Autodesk Inventor part; units mm, degrees
ref_plane "YZ Plane" through (0, 0, 0) normal (1, 0, 0) x (0, 1, 0)
ref_plane "XZ Plane" through (0, 0, 0) normal (0, 1, 0) x (-1, 0, 0)
ref_plane "XY Plane" through (0, 0, 0) normal (0, 0, 1) x (1, 0, 0)
sketch "Sketch1" plane through (0, 0, 0) normal (0, 0, 1) x (1, 0, 0)
  circle A0 centre (0, 0) radius 12.7
  line L0 (-0.074, 12.6998) -> (-0.074, 15.8748) construction
  line L1 (-0.074, 15.8748) -> (1.5135, 15.8748)
  line L2 (1.5135, 15.8748) -> (1.5135, 12.6095)
  line L3 (-0.074, 15.8748) -> (-1.6615, 15.8748)
  line L4 (-1.6615, 15.8748) -> (-1.6615, 12.5909)
  line L5 (-14.5787, 6.4985) -> (-11.7347, 4.8566)
  line L6 (-13.7849, 7.8733) -> (-14.5787, 6.4985)
  line L7 (-13.7849, 7.8733) -> (-12.9912, 9.2482)
  line L8 (-12.9912, 9.2482) -> (-10.1634, 7.6155)
  line L9 (-12.9172, -9.3763) -> (-10.0733, -7.7343)
  line L10 (-13.711, -8.0014) -> (-12.9172, -9.3763)
  line L11 (-13.711, -8.0014) -> (-14.5047, -6.6266)
  line L12 (-14.5047, -6.6266) -> (-11.6769, -4.994)
  line L13 (1.6615, -15.8748) -> (1.6615, -12.5909)
  line L14 (0.074, -15.8748) -> (1.6615, -15.8748)
  line L15 (0.074, -15.8748) -> (-1.5135, -15.8748)
  line L16 (-1.5135, -15.8748) -> (-1.5135, -12.6095)
  line L17 (14.5787, -6.4985) -> (11.7347, -4.8566)
  line L18 (13.7849, -7.8733) -> (14.5787, -6.4985)
  line L19 (13.7849, -7.8733) -> (12.9912, -9.2482)
  line L20 (12.9912, -9.2482) -> (10.1634, -7.6155)
  line L21 (12.9172, 9.3763) -> (10.0733, 7.7343)
  line L22 (13.711, 8.0014) -> (12.9172, 9.3763)
  line L23 (13.711, 8.0014) -> (14.5047, 6.6266)
  line L24 (14.5047, 6.6266) -> (11.6769, 4.994)
  line L25 (0, 0) -> (0, 9.525) construction
  line L26 (0, 6.35) -> (1.5875, 6.35)
  line L27 (1.5875, 6.35) -> (1.5875, 9.3918)
  line L28 (0, 6.35) -> (-1.5875, 6.35)
  line L29 (-1.5875, 6.35) -> (-1.5875, 9.3918)
  line L30 (-6.293, 1.8002) -> (-8.9273, 3.3211)
  line L31 (-5.4993, 3.175) -> (-6.293, 1.8002)
  line L32 (-5.4993, 3.175) -> (-4.7055, 4.5498)
  line L33 (-4.7055, 4.5498) -> (-7.3398, 6.0707)
  line L34 (-4.7055, -4.5498) -> (-7.3398, -6.0707)
  line L35 (-5.4993, -3.175) -> (-4.7055, -4.5498)
  line L36 (-5.4993, -3.175) -> (-6.293, -1.8002)
  line L37 (-6.293, -1.8002) -> (-8.9273, -3.3211)
  line L38 (1.5875, -6.35) -> (1.5875, -9.3918)
  line L39 (0, -6.35) -> (1.5875, -6.35)
  line L40 (0, -6.35) -> (-1.5875, -6.35)
  line L41 (-1.5875, -6.35) -> (-1.5875, -9.3918)
  line L42 (6.293, -1.8002) -> (8.9273, -3.3211)
  line L43 (5.4993, -3.175) -> (6.293, -1.8002)
  line L44 (5.4993, -3.175) -> (4.7055, -4.5498)
  line L45 (4.7055, -4.5498) -> (7.3398, -6.0707)
  line L46 (4.7055, 4.5498) -> (7.3398, 6.0707)
  line L47 (5.4993, 3.175) -> (4.7055, 4.5498)
  line L48 (5.4993, 3.175) -> (6.293, 1.8002)
  line L49 (6.293, 1.8002) -> (8.9273, 3.3211)
  arc A1 (7.3398, 6.0707) -> (1.5875, 9.3918) centre (0, 0) ccw
  arc A2 (8.9273, -3.3211) -> (8.9273, 3.3211) centre (0, 0) ccw
  arc A3 (1.5875, -9.3918) -> (7.3398, -6.0707) centre (0, 0) ccw
  arc A4 (-7.3398, -6.0707) -> (-1.5875, -9.3918) centre (0, 0) ccw
  arc A5 (-1.5875, 9.3918) -> (-7.3398, 6.0707) centre (0, 0) ccw
  arc A6 (-8.9273, 3.3211) -> (-8.9273, -3.3211) centre (0, 0) ccw
  dimension "outerDiameter" = 25.4
  dimension "splineHeight" = 3.175
  dimension "splineWidth" = 3.175
  dimension "d16" = 360
  dimension "d20" = 3.175
  dimension "d21" = 3.175
  dimension "d24" = 360
extrude "Extrusion4" add sketch "Sketch1" against normal blind 50.8
equation "\"d20\" = splineHeight"
equation "\"d21\" = splineWidth"
properties part number "outerShaft" material "PET Plastic"
Geometry: final body of the model. Coordinates: model frame, mm. A direction names the side the tool comes from. Round coordinates to 2 decimals unless told otherwise and drop trailing zeros. Order: outer loops, then holes, each group sorted by start corner. A loop starts at its lowest first (then second) coordinate and runs counter-clockwise, first axis right, second up. Notation, with made-up numbers: (40.5, -15) -> (57.5, -15) arc R15 cw to (57.5, -8) -> close; hole circle Ø6 at (61.25, 76.25). An arc over 180 degrees is marked (long way). Use CSV: the item, a comma, the result in double quotes. Start each with the question number.
1) Section A-A (x = -2.25). Return the cut outline in (y, z).
2) First-contact query: pin 1 Ø2 at (y, z) = (11, -23) entering from +X; pin 2 Ø3 at (y, z) = (-7.5, -29) entering from +X; pin 3 Ø3.5 at (y, z) = (-14.5, -16.5) entering from -X. Flat tips, straight axial feed; report the tip coordinate or a pass-through.
3) Material intervals for line 1 along Y through (x, z) = (1.25, -41.5); line 2 along X through (y, z) = (7.5, -44); line 3 along X through (y, z) = (8.5, -7), sorted ascending. Write a range as from..to.
4) Draft query along X for faces 5 (the face through (-1.662, 14, -25)), 6 (the face through (13.18, -5.69, -25.04)), 7 (the face through (1.588, -8, -25)). Return one class per face: +X half, -X half, draft (parallel to the pull), parting line (faces both ways), or undercut.
5) Set-up query: faces 1 (the face through (0, 6.35, -25)), 2 (the face through (13.11, 5.82, -25.04)), 3 (the face through (6.35, 11, -25.04)), 4 (the face through (6.35, -11, -25.04)). Return all of +Z, -Z, +X, -X, +Y, -Y with unobstructed straight access to the full face (end or side cutting, diameter ignored); none if empty.
6) Section B-B (y = 12). Return the cut outline in (x, z).
7) Section C-C (x = -11). Return the cut outline in (y, z), and give its area (3 significant figures).
Returned:
1,outline,"(-12.5, -50.8) -> (-9.26, -50.8) -> (-9.26, 0) -> (-12.5, 0) -> close; (9.26, -50.8) -> (12.5, -50.8) -> (12.5, 0) -> (9.26, 0) -> close"
2,pin 1,"stops at x = 7.83"
2,pin 2,"stops at x = 14.58"
2,pin 3,"stops at x = -1.51"
3,line 1,"y = -15.87..-6.35, 6.35..15.87"
3,line 2,"x = -14..-5.87, -1.59..1.59, 5.87..14"
3,line 3,"x = -13.42..-11.7, -9.44..-4.3, -1.59..1.59, 4.3..9.44, 11.4..13.42"
4,face 5,"-X half"
4,face 6,"+X half"
4,face 7,"undercut"
5,face 1,"+Z, -Z"
5,face 2,"+Z, -Z, +X"
5,face 3,"+Z, -Z, +Y"
5,face 4,"+Z, -Z, -Y"
6,outline,"(-4.16, -50.8) -> (4.16, -50.8) -> (4.16, 0) -> (-4.16, 0) -> close"
7,outline,"(-8.27, -50.8) -> (8.1, -50.8) -> (8.1, 0) -> (-8.27, 0) -> close"
7,area,"831 mm²"
